Can you work these out from the model? Positions are in its coordinate system, mm. A direction names the side the tool comes from. Round coordinates to 2 decimals unless told otherwise and drop trailing zeros. Order: outer loops, then holes, each group sorted by start corner. A loop starts at its lowest first (then second) coordinate and runs counter-clockwise, first axis right, second up. Notation, with made-up numbers: (-15, 23.5) -> (17, 23.5) arc R32 ccw to (17, 62.5) -> close; hole circle Ø9 at (-34.75, 65). An arc over 180 degrees is marked (long way). One line per item, written item: value.
```python
from build123d import *

# Parameters (mm, degrees)
PAD_DEPTH       = 16
POCKET_DEPTH    = 14
SKETCH002_R     = 2.1
POCKET001_DEPTH = 100
SKETCH003_R     = 2.1
POCKET002_DEPTH = 100
FILLET_R        = 0.2
FILLET001_R     = 0.2
FILLET002_R     = 0.2


with BuildPart() as part:
    # Sketch → Pad (new body)
    with BuildSketch(Plane.XY):
        Polygon((-5, 28), (5, 28), (5, 24), (24, 5), (28, 5), (28, -5), (24, -5), (5, -24), (5, -28), (-5, -28), (-5, -24), (-24, -5), (-28, -5), (-28, 5), (-24, 5), (-5, 24), align=None)
    extrude(amount=PAD_DEPTH)

    # Sketch001 (on Face18 of Pad) → Pocket (cut)
    with BuildSketch(Plane.XY.offset(16)):
        Polygon((5, 20), (-5, 20), (-20, 5), (-20, -5), (-5, -20), (5, -20), (20, -5), (20, 5), align=None)
    extrude(amount=-POCKET_DEPTH, mode=Mode.SUBTRACT)

    # Sketch002 (on Face17 of Pocket) → Pocket001 (cut)
    with BuildSketch(Plane.XZ.offset(28)):
        with Locations((0, 9)):
            Circle(SKETCH002_R)
    extrude(amount=-POCKET001_DEPTH, mode=Mode.SUBTRACT)

    # Sketch003 (on Face13 of Pocket001) → Pocket002 (cut)
    with BuildSketch(Plane.YZ.offset(28)):
        with Locations((0, 9)):
            Circle(SKETCH003_R)
    extrude(amount=-POCKET002_DEPTH, mode=Mode.SUBTRACT)

    # Fillet
    fillet_edges = [part.edges().sort_by_distance(p)[0] for p in [
        (28, 0, 16),
        (26, 5, 16),
        (14.5, 14.5, 16),
        (26, -5, 16),
        (14.5, -14.5, 16),
        (5, -26, 16),
        (0, -28, 16),
        (-5, -26, 16),
        (-14.5, -14.5, 16),
        (-26, -5, 16),
        (-28, 0, 16),
        (-26, 5, 16),
        (-14.5, 14.5, 16),
        (-5, 26, 16),
        (0, 28, 16),
        (5, 26, 16),
    ]]
    fillet(fillet_edges, radius=FILLET_R)

    # Fillet001
    fillet001_edges = [part.edges().sort_by_distance(p)[0] for p in [
        (12.5, 12.5, 16),
        (20, 0, 16),
        (12.5, -12.5, 16),
        (0, -20, 16),
        (-12.5, -12.5, 16),
        (-20, 0, 16),
        (-12.5, 12.5, 16),
        (0, 20, 16),
    ]]
    fillet(fillet001_edges, radius=FILLET001_R)

    # Fillet002
    fillet002_edges = [part.edges().sort_by_distance(p)[0] for p in [
        (0, 28, 0),
        (-14.5, 14.5, 0),
        (-5, 26, 0),
        (5, 26, 0),
        (14.5, 14.5, 0),
        (26, 5, 0),
        (28, 0, 0),
        (26, -5, 0),
        (14.5, -14.5, 0),
        (5, -26, 0),
        (0, -28, 0),
        (-5, -26, 0),
        (-14.5, -14.5, 0),
        (-26, -5, 0),
        (-28, 0, 0),
        (-26, 5, 0),
    ]]
    fillet(fillet002_edges, radius=FILLET002_R)


solid = part.part
```
Q1. We'd pull the mould along Y, two halves only. Please class faces 1 (the face through (14.591, 14.324, 15.943)), 2 (the face through (-14, -15, 8)), 3 (the face through (-28, 0, 6)), 4 (the face through (13, 12, 9)): released by +Y, released by -Y, zero draft, split by the parting line, or undercut.
Answers below:
face 1: released by +Y
face 2: released by -Y
face 3: zero draft
face 4: undercut
Q2. I want a section at D-D on z = 9. Give the number of separate pieces and of enclosed holes in the cut face, plus the area to 3 significant figures.
Answers below:
separate pieces: 4
enclosed holes: 0
area: 458 mm^2
Q3. I want a section at C-C on z = 2.75. List the corners of the cut face in (x, y) for me, plus the area to 3 significant figures.
Answers below:
outline: (-28, -5) -> (-24, -5) -> (-5, -24) -> (-5, -28) -> (5, -28) -> (5, -24) -> (24, -5) -> (28, -5) -> (28, 5) -> (24, 5) -> (5, 24) -> (5, 28) -> (-5, 28) -> (-5, 24) -> (-24, 5) -> (-28, 5) -> close; hole (-20, -5) -> (-5, -20) -> (5, -20) -> (20, -5) -> (20, 5) -> (5, 20) -> (-5, 20) -> (-20, 5) -> close
area: 592 mm^2
Q4. I want a section at A-A on x = 0. List the corners of the cut face in (y, z) for me.
Answers below:
outline: (-28, 0.2) arc R0.2 ccw to (-27.8, 0) -> (27.8, 0) arc R0.2 ccw to (28, 0.2) -> (28, 6.9) -> (20, 6.9) -> (20, 2) -> (-20, 2) -> (-20, 6.9) -> (-28, 6.9) -> close; (-28, 11.1) -> (-20, 11.1) -> (-20, 15.8) arc R0.2 ccw to (-20.2, 16) -> (-27.8, 16) arc R0.2 ccw to (-28, 15.8) -> close; (20, 11.1) -> (28, 11.1) -> (28, 15.8) arc R0.2 ccw to (27.8, 16) -> (20.2, 16) arc R0.2 ccw to (20, 15.8) -> close
Q5. Please list where these lines run through material, in increasing order: line 1 along Z through (x, y) = (0, -22.5); line 2 along X through (y, z) = (-3.5, 6.25); line 3 along Z through (x, y) = (15, -8).
Answers below:
line 1: 0 to 6.9, 11.1 to 16
line 2: -28 to -20, 20 to 28
line 3: 0 to 2
Q6. Will these pins go through, and if not, where does the flat tip stop? pin 1 Ø1.2 at (x, z) = (26.5, 5) entering from +Y; pin 2 Ø6 at (x, z) = (9.5, 12) entering from +Y; pin 3 Ø1.2 at (x, z) = (25, 9) entering from -Y.
Answers below:
pin 1: y = 5
pin 2: y = 22.5
pin 3: y = -5
Q7. On a 3-axis mill with a long thin cutter (end or side, diameter ignored), from which of +Z, -Z, +X, -X, +Y, -Y can I reach the whole of each face in a straight line? I mean faces 5 (the face through (28, 0, 6)), 6 (the face through (0, -28, 6)), 7 (the face through (5, -26, 8)), 8 (the face through (20, -2.3, 9)), 9 (the face through (5, 26, 8)). Say none if no direction works.
Answers below:
face 5: +Z, -Z, +X, +Y, -Y
face 6: +Z, -Z, +X, -X, -Y
face 7: +Z, -Z, +X, -Y
face 8: +Z
face 9: +Z, -Z, +X, +Y
